```python
from build123d import *

# Parameters (mm, degrees)
SKETCH_1_W            = 42.4
SKETCH_1_H            = 21.6
SKETCH_1_R            = 1.1
EXTRUDE_1_DEPTH       = 1
SKETCH_2_W            = 18
SKETCH_2_H            = 14
SKETCH_2_W_2          = 8
SKETCH_2_H_2          = 8.9
EXTRUDE_2_DEPTH       = 3
FILLET_1_R            = 1
SKETCH_2_3_W          = 18
SKETCH_2_3_H          = 6.1
EXTRUDE_3_DEPTH       = 1
CUT_EXTRUDE_1_DEPTH   = 7.7
SKETCH_4_W            = 18
SKETCH_4_H            = 14
SKETCH_4_W_2          = 16
SKETCH_4_H_2          = 12
CUT_EXTRUDE_1_2_DEPTH = 2


with BuildPart() as part:
    # 草图1 → 凸台-拉伸1 (new body)
    with BuildSketch(Plane(origin=(0, 0, 0), x_dir=(1, 0, 0), z_dir=(0, 1, 0))):
        Rectangle(SKETCH_1_W, SKETCH_1_H)
        with Locations((-18, 0)):
            Circle(SKETCH_1_R, mode=Mode.SUBTRACT)
        with Locations((19.2, 8.8)):
            Circle(SKETCH_1_R, mode=Mode.SUBTRACT)
        with Locations((19.2, -8.8)):
            Circle(SKETCH_1_R, mode=Mode.SUBTRACT)
    extrude(amount=EXTRUDE_1_DEPTH)

    # 草图2 → 凸台-拉伸2 (add)
    with BuildSketch(Plane(origin=(0, 1, 0), x_dir=(1, 0, 0), z_dir=(0, 1, 0))):
        with Locations((-2.04, -2.3)):
            Rectangle(SKETCH_2_W, SKETCH_2_H)
        with Locations((17, -2.15)):
            Rectangle(SKETCH_2_W_2, SKETCH_2_H_2)
    extrude(amount=EXTRUDE_2_DEPTH)

    # 圆角1
    fillet_1_edges = [part.edges().sort_by_distance(p)[0] for p in [
        (17, 4, -2.3),
        (17, 4, 6.6),
    ]]
    fillet(fillet_1_edges, radius=FILLET_1_R)

    # 草图2<3> → 凸台-拉伸3 (add)
    with BuildSketch(Plane(origin=(0, 1, 0), x_dir=(1, 0, 0), z_dir=(0, 1, 0))):
        with Locations((-2.04, 7.75)):
            Rectangle(SKETCH_2_3_W, SKETCH_2_3_H)
    extrude(amount=EXTRUDE_3_DEPTH)

    # 草图3 → Cut-Extrude 1 (cut)
    with BuildSketch(Plane(origin=(21, 0, 0), x_dir=(0, 0, -1), z_dir=(1, 0, 0))):
        with BuildLine():
            Line((1.3, 3.7), (-5.6, 3.7))
            ThreePointArc((-5.6, 3.7), (-6.094974747, 3.494974747), (-6.3, 3))
            Line((-6.3, 3), (-6.3, 1.3))
            Line((-6.3, 1.3), (2, 1.3))
            Line((2, 1.3), (2, 3))
            ThreePointArc((2, 3), (1.794974747, 3.494974747), (1.3, 3.7))
        make_face()
    extrude(amount=-CUT_EXTRUDE_1_DEPTH, mode=Mode.SUBTRACT)

    # 草图4 → Cut-Extrude 1 2 (cut)
    with BuildSketch(Plane(origin=(0, 4, 0), x_dir=(1, 0, 0), z_dir=(0, 1, 0))):
        with Locations((-2.04, -2.3)):
            Rectangle(SKETCH_4_W, SKETCH_4_H)
        with Locations((-2.04, -2.3)):
            Rectangle(SKETCH_4_W_2, SKETCH_4_H_2, mode=Mode.SUBTRACT)
    extrude(amount=-CUT_EXTRUDE_1_2_DEPTH, mode=Mode.SUBTRACT)


solid = part.part
```
Here's how the part is built. I have some questions about the finished solid (model axes, mm). A direction names the side the tool comes from. Round coordinates to 2 decimals unless told otherwise and drop trailing zeros. Write each loop counter-clockwise with the first axis right and the second up, starting at its lowest first coordinate (ties: lowest second). Pieces come first, ordered by that corner, then holes.
Q1. Please list where these lines run through material, in increasing order: probe 1 along Z at (x, y) = (19.2, 0.45); probe 2 along Z at (x, y) = (16.5, 1.65); probe 3 along X at (y, z) = (2.75, 4.25).
Q2. If we section it at C-C on y = 2.4: Write out the boundary of the cut face in (x, z).
Q3. If we section it at B-B on z = 0: Write out the boundary of the cut face in (x, y), plus the area to 3 significant figures.
Q4. Which directions (+Z, -Z, +X, -X, +Y, -Y) give clear straight access to the entire face, cutting with the end or side of a thin tool? Please do faces 1 (the flat face through (-2, 3, -3.7)), 2 (the flat face through (17, 2, -2.3)), 3 (the flat face through (-11.04, 1.5, -0.6)), 4 (the flat face through (13, 2, 2)), 5 (the flat face through (-2.2, 1.5, 9.3)).
Q5. If we section it at D-D on x = -18: Write out the boundary of the cut face in (y, z), plus the area to 3 significant figures.
Q6. Will these pins go through, and if not, where does the flat tip stop? P1, Ø1.6, axis at x = 17.5, y = 1.5, coming from the +Z side; P2, Ø1, axis at x = -15.5, z = -3.5, coming from the +Y side; P3, Ø1, axis at y = 3, z = 3.5, coming from the +X side; P4, Ø0.6, axis at x = 1, y = 2.5, coming from the +Z side.
Q7. If we mould it in two halves opening along Z, with no side actions, what happens to faces 6 (the flat face through (-0.3, 0.5, 10.8)), 7 (the flat face through (13.3, 3, 2)), 8 (the flat face through (9, 1, 0))? For each: +Z half, -Z half, draft (parallel to the pull), parting line (faces both ways), or undercut.
Q8. If we section it at A-A on x = 19.2: Write out the boundary of the cut face in (y, z), plus the area to 3 significant figures.
Answer below:
1. probe 1: z = -10.8 to -9.9, -7.7 to 7.7, 9.9 to 10.8
1. probe 2: z = -2.3 to -2, 6.3 to 6.6
1. probe 3: x = -10.04 to 5.96, 13 to 13.3
2. outline: (-10.04, -3.7) - (5.96, -3.7) - (5.96, 8.3) - (-10.04, 8.3) - close; (13, -2.3) - (21, -2.3) - (21, -2) - (13.3, -2) - (13.3, 6.3) - (21, 6.3) - (21, 6.6) - (13, 6.6) - close
3. outline: (-21.2, 0) - (-19.1, 0) - (-19.1, 1) - (-21.2, 1) - close; (-16.9, 0) - (21.2, 0) - (21.2, 1) - (21, 1) - (21, 1.3) - (13.3, 1.3) - (13.3, 3.7) - (21, 3.7) - (21, 4) - (13, 4) - (13, 1) - (6.96, 1) - (6.96, 2) - (5.96, 2) - (5.96, 4) - (-10.04, 4) - (-10.04, 2) - (-11.04, 2) - (-11.04, 1) - (-16.9, 1) - close
3. area: 95.7 mm2
4. face 1: -Z, +X, -X, +Y
4. face 2: -Z, +X, +Y
4. face 3: +Z, -Z, -X, +Y
4. face 4: +Z, -Z, +Y
4. face 5: +Z, +X, -X, +Y
5. outline: (0, -10.8) - (1, -10.8) - (1, -1.1) - (0, -1.1) - close; (0, 1.1) - (1, 1.1) - (1, 10.8) - (0, 10.8) - close
5. area: 19.4 mm2
6. P1: stops at z = 10.8
6. P2: stops at y = 1
6. P3: stops at x = 13.3
6. P4: stops at z = 8.3
7. face 6: +Z half
7. face 7: undercut
7. face 8: draft
8. outline: (0, -10.8) - (1, -10.8) - (1, -9.9) - (0, -9.9) - close; (0, -7.7) - (1, -7.7) - (1, -2.3) - (3, -2.3) arc R1 ccw to (4, -1.3) - (4, 5.6) arc R1 ccw to (3, 6.6) - (1, 6.6) - (1, 7.7) - (0, 7.7) - close; (0, 9.9) - (1, 9.9) - (1, 10.8) - (0, 10.8) - close; hole (1.3, -2) - (3, -2) arc R0.7 ccw to (3.7, -1.3) - (3.7, 5.6) arc R0.7 ccw to (3, 6.3) - (1.3, 6.3) - close
8. area: 23.8 mm2
